from build123d import *

# Parameters (mm, degrees)
BASPROSKE_W             = 48
BASPROSKE_H             = 42
TOOTHCUT_DEPTH          = 77.367532368
TEETHCUTS_COUNT         = 40
TEETHCUTS_ANGLE         = 351
BORSKE_R                = 32.5
BORE_DEPTH              = 50.0000508
CUT_EXTRUDE1_DEPTH      = 77.274548253
CUT_EXTRUDE1_DEPTH_BACK = 77.274548253
SKETCH1_R               = 34.65
CUT_EXTRUDE2_DEPTH      = 77.274548253
CUT_EXTRUDE2_DEPTH_BACK = 77.274548253
SKETCH2_W               = 102.897600885
SKETCH2_H               = 48.377080865
BOSS_EXTRUDE1_START     = -12.28816495
BOSS_EXTRUDE1_DEPTH     = 12.28816495
SKETCH4_R               = 3.25
CUT_EXTRUDE3_DEPTH      = 84.350383201
MIRROR3_COPY_1_SKETCH_R = 3.25
MIRROR3_COPY_1_DEPTH    = 84.350383201
FILLET1_R               = 3


with BuildPart() as part:
    # BasProSke → Base-Revolve (revolve)
    with BuildSketch(Plane(origin=(0, 0, 0), x_dir=(1, 0, 0), z_dir=(0, 1, 0)), mode=Mode.PRIVATE) as base_revolve_sk:
        with Locations((24, 21)):
            Rectangle(BASPROSKE_W, BASPROSKE_H)
    revolve(base_revolve_sk.sketch.rotate(Axis((-10, 0, 0), (1, 0, 0)), 180), axis=Axis((-10, 0, 0), (1, 0, 0)))

    # TooCutSke → ToothCut (cut, through all)
    with BuildSketch(Plane(origin=(0, 0, 0), x_dir=(0, 0, -1), z_dir=(1, 0, 0))):
        with BuildLine():
            ThreePointArc((0.882812088, 37.488606854), (0, 37.499), (-0.882812088, 37.488606854))
            ThreePointArc((-0.882812088, 37.488606854), (-1.612748684, 39.782000434), (-2.678427154, 41.939960338))
            ThreePointArc((-2.678427154, 41.939960338), (0, 42.0254), (2.678427154, 41.939960338))
            ThreePointArc((2.678427154, 41.939960338), (1.612748684, 39.782000434), (0.882812088, 37.488606854))
        make_face()
    toothcut = extrude(amount=TOOTHCUT_DEPTH, mode=Mode.SUBTRACT)

    # TeethCuts: ToothCut ×40 about axis
    teethcuts_axis = Axis((-10, 0, 0), (1, 0, 0))
    for i in range(1, TEETHCUTS_COUNT):
        add(toothcut.rotate(teethcuts_axis, i * TEETHCUTS_ANGLE / (TEETHCUTS_COUNT - 1)), mode=Mode.SUBTRACT)

    # BorSke → Bore (cut, symmetric)
    with BuildSketch(Plane(origin=(0, 0, 0), x_dir=(0, 0, -1), z_dir=(1, 0, 0))):
        with Locations(Location((0, 0, 0), (0, 0, 180))):
            Circle(BORSKE_R)
    extrude(amount=BORE_DEPTH, both=True, mode=Mode.SUBTRACT)

    # Sketch1 → Cut-Extrude1 (cut, two sides: drawn at the far end of the back side and taken through both)
    with BuildSketch(Plane.ZY.offset(-CUT_EXTRUDE1_DEPTH_BACK)):
        Circle(SKETCH1_R)
    extrude(amount=CUT_EXTRUDE1_DEPTH + CUT_EXTRUDE1_DEPTH_BACK, mode=Mode.SUBTRACT)

    # Sketch2 → Cut-Extrude2 (cut, two sides: drawn at the far end of the back side and taken through both)
    with BuildSketch(Plane(origin=(48, 0, 0), x_dir=(0, 0, -1), z_dir=(1, 0, 0)).offset(-CUT_EXTRUDE2_DEPTH_BACK)):
        with Locations((0.168316686, 24.188540433)):
            Rectangle(SKETCH2_W, SKETCH2_H)
    extrude(amount=CUT_EXTRUDE2_DEPTH + CUT_EXTRUDE2_DEPTH_BACK, mode=Mode.SUBTRACT)

    # Sketch3 → Boss-Extrude1 (add)
    with BuildSketch(Plane(origin=(48, 0, 0), x_dir=(0, 0, -1), z_dir=(1, 0, 0)).offset(BOSS_EXTRUDE1_START)):
        with BuildLine():
            Line((34.65, 0), (57.182596138, 0))
            Line((57.182596138, 0), (57.182596138, -6.740320101))
            Line((57.182596138, -6.740320101), (43.278498338, -6.740320101))
            ThreePointArc((43.278498338, -6.740320101), (0, -43.800232116), (-43.278498338, -6.740320101))
            Line((-43.278498338, -6.740320101), (-57.182596138, -6.740320101))
            Line((-57.182596138, -6.740320101), (-57.182596138, 0))
            Line((-57.182596138, 0), (-34.65, 0))
            ThreePointArc((-34.65, 0), (0, -34.65), (34.65, 0))
        make_face()
    boss_extrude1 = extrude(amount=BOSS_EXTRUDE1_DEPTH)

    # Mirror1: Boss-Extrude1 across plane
    add(boss_extrude1.mirror(Plane(origin=(24, 0, 0), x_dir=(0, 0, 1), z_dir=(1, 0, 0))))

    # Sketch4 → Cut-Extrude3 (cut, symmetric)
    with BuildSketch(Plane.XZ.offset(6.740320101)):
        with Locations(Location((41.855917525, 50.230547238, 0), (0, 0, 270))):
            Circle(SKETCH4_R)
    cut_extrude3 = extrude(amount=CUT_EXTRUDE3_DEPTH, both=True, mode=Mode.SUBTRACT)

    # Mirror2: Cut-Extrude3 across plane
    add(cut_extrude3.mirror(Plane.XY), mode=Mode.SUBTRACT)

    # Mirror3: Cut-Extrude3 across plane
    add(cut_extrude3.mirror(Plane(origin=(24, 0, 0), x_dir=(0, 0, 1), z_dir=(1, 0, 0))), mode=Mode.SUBTRACT)

    # Mirror3 copy 1 sketch → Mirror3 copy 1 (cut, symmetric)
    with BuildSketch(Plane(origin=(48, -6.740320101, 0), x_dir=(-1, 0, 0), z_dir=(0, -1, 0))):
        with Locations(Location((41.855917525, 50.230547238, 0), (0, 0, 270))):
            Circle(MIRROR3_COPY_1_SKETCH_R)
    extrude(amount=MIRROR3_COPY_1_DEPTH, both=True, mode=Mode.SUBTRACT)

    # Fillet1
    fillet1_edges = [part.edges().sort_by_distance(p)[0] for p in [
        (0, -3.37016005, -57.182596138),
        (0, -3.37016005, 57.182596138),
        (12.28816495, -3.37016005, 57.182596138),
        (12.28816495, -3.37016005, -57.182596138),
        (35.71183505, -3.37016005, -57.182596138),
        (35.71183505, -3.37016005, 57.182596138),
        (48, -3.37016005, 57.182596138),
        (48, -3.37016005, -57.182596138),
    ]]
    fillet(fillet1_edges, radius=FILLET1_R)


solid = part.part
Read the model definition and answer for the solid it produces. Units are mm, in the model's axes. A direction names the side the tool comes from. Coordinates: 2 decimals unless noted, no trailing zeros. Order: outer loops, then holes, each group sorted by start corner. A loop starts at its lowest first (then second) coordinate and runs counter-clockwise, first axis right, second up. Notation, with made-up numbers: (76.5, 35.5) -> (93.5, 35.5) arc R20 cw to (93.5, 60.5) -> close; hole circle Ø11 at (40.25, 63.25). An arc over 180 degrees is marked (long way). Answer as a JSON object with one key per item and string values.
1) A tool of negligible diameter and unlimited length cuts with its end or side. For faces 4 (the face through (23.836, -33.151, -22.083)), 5 (the face through (23.84, -7.83, -39.06)), 6 (the face through (23.84, -7.79, 39)), from which of +Z, -Z, +X, -X, +Y, -Y can it reach the whole face along a straight path? Write none if from no direction.
Model answer:
{"face 4": "none", "face 5": "-Z", "face 6": "+Z"}
2) A cutting plane is placed at C-C, the plane z = -50. Determine the outline of the cut face in (x, y), plus the area to 3 significant figures.
Model answer:
{"outline": "(0, -6.74) -> (2.9, -6.74) -> (2.9, 0) -> (0, 0) -> close; (9.39, -6.74) -> (12.29, -6.74) -> (12.29, 0) -> (9.39, 0) -> close; (35.71, -6.74) -> (38.61, -6.74) -> (38.61, 0) -> (35.71, 0) -> close; (45.1, -6.74) -> (48, -6.74) -> (48, 0) -> (45.1, 0) -> close", "area": "78.2 mm²"}
3) The mould has two halves that part along Y. Classify faces 1 (the face through (23.836, -29.227, 26.971)), 2 (the face through (36.614, -3.417, -56.327)), 3 (the face through (6.23, -43.79, -0.87)): released by +Y, released by -Y, zero draft, split by the parting line, or undercut.
Model answer:
{"face 1": "undercut", "face 2": "zero draft", "face 3": "released by -Y"}
4) A cutting plane is placed at B-B, the plane x = 7.5. Determine the outline of the cut face in (y, z), plus the area to 3 significant figures.
Model answer:
{"outline": "(-6.74, -57.18) -> (0, -57.18) -> (0, -53.18) -> (-6.74, -53.18) -> close; (-6.74, -47.28) -> (0, -47.28) -> (0, -34.65) arc R34.65 cw to (0, 34.65) -> (0, 47.28) -> (-6.74, 47.28) -> (-6.74, 43.28) arc R43.8 ccw to (-6.74, -43.28) -> close; (-6.74, 53.18) -> (0, 53.18) -> (0, 57.18) -> (-6.74, 57.18) -> close", "area": "1,230 mm²"}
5) A cutting plane is placed at A-A, the plane y = -24.5. Determine the outline of the cut face in (x, z), plus the area to 3 significant figures.
Model answer:
{"outline": "(0, -36.31) -> (12.29, -36.31) -> (12.29, -31.12) -> (35.71, -31.12) -> (35.71, -36.31) -> (48, -36.31) -> (48, -24.5) -> (0, -24.5) -> close; (0, 24.5) -> (48, 24.5) -> (48, 36.31) -> (35.71, 36.31) -> (35.71, 31.12) -> (12.29, 31.12) -> (12.29, 36.31) -> (0, 36.31) -> close", "area": "890 mm²"}
6) A cutting plane is placed at D-D, the plane z = -20. Determine the outline of the cut face in (x, y).
Model answer:
{"outline": "(0, -38.97) -> (12.29, -38.97) -> (12.29, -35.13) -> (35.71, -35.13) -> (35.71, -38.97) -> (48, -38.97) -> (48, -28.3) -> (0, -28.3) -> close"}
7) Consider line 1 along Z through (x, y) = (33.5, -40); line 2 along Z through (x, y) = (13.5, -30); line 3 along Z through (x, y) = (38.5, -13.5). Determine where each line is inside the solid, lowest interval first. Write a range as from..to.
Model answer:
{"line 1": "z = -10.56..-8.44, -4.52..-1.7, 1.7..4.52, 8.44..10.56", "line 2": "z = -27.28..-22.97, -22.5..-17.34, 17.34..22.5, 22.97..27.28", "line 3": "z = -41.67..-31.91, 31.91..41.67"}
8) Each of these flat-tipped pins is pushed along its axis until it touches: pin 1 (10 mm diameter, centred on x = 16, z = -33, fed in from -Y); pin 2 (5 mm diameter, centred on x = 28, y = -8.5, fed in from -Z); pin 3 (6 mm diameter, centred on x = 6.5, z = -48, fed in from -Y). Where does it stop, or does it pass through?
Model answer:
{"pin 1": "stops at y = -32.24", "pin 2": "stops at z = -40.98", "pin 3": "stops at y = -6.74"}
